```python
from build123d import *

# Parameters (mm, degrees)
F0_R      = 10
F0_R_2    = 3.05
F1_DEPTH  = 12.5
F3_R      = 7.45
F4_DEPTH  = 33.3293554535
F5_R      = 2.975
F6_DEPTH  = 39.3287836491
F7_R      = 2
F8_R      = 1.1303
F9_DEPTH  = 12.5
F11_R     = 2.5
F12_DEPTH = 25
F13_W     = 67.0658163726
F13_H     = 16.5084768087
F14_DEPTH = 12.5


with BuildPart() as f1:
    # F0 (on Top) → F1 (new body, symmetric)
    with BuildSketch(Plane.XY):
        Circle(F0_R)
        Circle(F0_R_2, mode=Mode.SUBTRACT)
    extrude(amount=F1_DEPTH, both=True)

    # F3 (on offset) → F4 (join, through all)
    with BuildSketch(Plane.YZ.offset(40)):
        Circle(F3_R)
    extrude(amount=-F4_DEPTH)

    # F5 (on face) → F6 (cut, through all)
    with BuildSketch(Plane.YZ.offset(40)):
        Circle(F5_R)
    extrude(amount=-F6_DEPTH, mode=Mode.SUBTRACT)

    # F7
    f7_edges = [f1.edges().sort_by_distance(p)[0] for p in [
        (40, -7.45, 0),
    ]]
    fillet(f7_edges, radius=F7_R)

    # F8 (on Front) → F9 (cut, symmetric)
    with BuildSketch(Plane.XZ):
        with Locations((-6.5, -8)):
            Circle(F8_R)
        with Locations((6.5, -8)):
            Circle(F8_R)
        with Locations((-6.5, 8)):
            Circle(F8_R)
        with Locations((6.5, 8)):
            Circle(F8_R)
    extrude(amount=F9_DEPTH, both=True, mode=Mode.SUBTRACT)

    # F11 (on offset) → F12 (cut)
    with BuildSketch(Plane.XZ.offset(4.7)):
        with Locations((-6.5, 8)):
            Circle(F11_R)
        with Locations((6.5, 8)):
            Circle(F11_R)
        with Locations((-6.5, -8)):
            Circle(F11_R)
        with Locations((6.5, -8)):
            Circle(F11_R)
    extrude(amount=F12_DEPTH, mode=Mode.SUBTRACT)

    # F13 (on Top) → F14 (cut, symmetric)
    with BuildSketch(Plane.XY):
        with Locations((14.590991661, 8.2542384043)):
            Rectangle(F13_W, F13_H)
    extrude(amount=F14_DEPTH, both=True, mode=Mode.SUBTRACT)


solid = f1.part
```
Source: CAD feature listing. Evaluate the final solid. Frame: model axes, mm. A direction names the side the tool comes from. Give positions to 0.01 mm unless a question says otherwise; leave off trailing zeros. Order: outer loops, then holes, each group sorted by start corner. A loop starts at its lowest first (then second) coordinate and runs counter-clockwise, first axis right, second up.
(1) Section query B-B (y = -1). State how many separate pieces and enclosed holes the cut face has, plus the area to 3 significant figures.
(2) Access query for faces 1 (the face through (5, -4.7, 8)), 2 (the face through (20.609, -2.974, 0.065)), 3 (the face through (-5.42, -2.38, 8.34)). Directions: +Z, -Z, +X, -X, +Y, -Y. A direction counts if a zero-diameter tool reaches every point of the face in a straight line with its end or side. Return the directions, or none.
(3) Contact query for flat-ended pins moving along their axis: P1, Ø1, axis at y = -8, z = -3.5, coming from the +X side; P2, Ø1.4, axis at x = -6.5, z = 8.5, coming from the -Y side; P3, Ø2, axis at x = 19.5, z = 1, coming from the -Y side. Output: stop coordinate, or through.
(4) Pull-direction query (Z, two-part tool) for faces 4 (the face through (7.58, -2.38, 8.34)), 5 (the face through (-0.07, -3.05, -0.18)), 6 (the face through (22.55, -7.45, 0.16)); classes: +Z half, -Z half, draft (parallel to the pull), parting line (faces both ways), or undercut.
(5) Section query C-C (x = 1.5). Return the cut outline in (y, z) (3 decimals), plus the area to 3 significant figures.
(6) Material intervals for line 1 along Z through (x, y) = (6.5, -7.5); line 2 along Z through (x, y) = (-7, -2.5); line 3 along X through (y, z) = (-8.1, 8), sorted ascending.
(7) Section query A-A (x = -6.5). Return the cut outline in (y, z).
Outcome:
1. separate pieces: 3
1. enclosed holes: 4
1. area: 571 mm2
2. face 1: -Y
2. face 2: +X, +Y
2. face 3: +Y, -Y
3. P1: stops at x = 6.61
3. P2: stops at y = -4.7
3. P3: stops at y = -7.45
4. face 4: undercut
4. face 5: draft
4. face 6: parting line
5. outline: (-9.887, -12.5) - (-2.656, -12.5) - (-2.656, -1.341) arc R2.975 cw to (-2.656, 1.341) - (-2.656, 12.5) - (-9.887, 12.5) - close
5. area: 180 mm2
6. line 1: z = -12.5 to -10.5, -5.5 to 5.5, 10.5 to 12.5
6. line 2: z = -12.5 to -9.01, -6.99 to 6.99, 9.01 to 12.5
6. line 3: x = -4 to 4
7. outline: (-7.6, -12.5) - (0, -12.5) - (0, -9.13) - (-4.7, -9.13) - (-4.7, -10.5) - (-7.6, -10.5) - close; (-7.6, -5.5) - (-4.7, -5.5) - (-4.7, -6.87) - (0, -6.87) - (0, 6.87) - (-4.7, 6.87) - (-4.7, 5.5) - (-7.6, 5.5) - close; (-7.6, 10.5) - (-4.7, 10.5) - (-4.7, 9.13) - (0, 9.13) - (0, 12.5) - (-7.6, 12.5) - close
